from build123d import *

# Parameters (mm, degrees)
F0_W        = 127
F0_H        = 25.4
F1_DEPTH    = 3.175
F2_W        = 63.5
F2_H        = 7.9375
F3_DEPTH    = 25.4
F4_T1_DEPTH = 6.35
F5_R        = 5.08
F6_R        = 3.175
F7_DEPTH    = 25.4


# Not quite as in the source:
# - a fillet or chamfer that OpenCascade refuses, or shapes differently, is made with other operations: its cross-section is extruded or revolved along the edge and cut away or added


with BuildPart() as f1:
    # F0 (on Top) → F1 (new body, symmetric)
    with BuildSketch(Plane.XY):
        Rectangle(F0_W, F0_H)
    extrude(amount=F1_DEPTH, both=True)

    # F2 (on face) → F3 (cut)
    with BuildSketch(Plane.XY.offset(3.175)):
        with Locations((0, 8.73125)):
            Rectangle(F2_W, F2_H)
        with Locations((0, -8.73125)):
            Rectangle(F2_W, F2_H)
    extrude(amount=-F3_DEPTH, mode=Mode.SUBTRACT)

    # F4: fillet of radius 38.1 on 4 edges, made by hand

    # F4_s2 → F4_t1 (join)
    with BuildSketch(Plane.XY.offset(-3.175)):
        with BuildLine():
            ThreePointArc((-31.75, 12.7), (-20.7694028252, 6.8014320042), (-8.4726807009, 4.7625))
            Line((-8.4726807009, 4.7625), (-31.75, 4.7625))
            Line((-31.75, 4.7625), (-31.75, 12.7))
        make_face()
        with BuildLine():
            ThreePointArc((8.4726807009, 4.7625), (20.7694028252, 6.8014320042), (31.75, 12.7))
            Line((31.75, 12.7), (31.75, 4.7625))
            Line((31.75, 4.7625), (8.4726807009, 4.7625))
        make_face()
        with BuildLine():
            ThreePointArc((31.75, -12.7), (20.7694028252, -6.8014320042), (8.4726807009, -4.7625))
            Line((8.4726807009, -4.7625), (31.75, -4.7625))
            Line((31.75, -4.7625), (31.75, -12.7))
        make_face()
        with BuildLine():
            ThreePointArc((-31.75, -12.7), (-20.7694028252, -6.8014320042), (-8.4726807009, -4.7625))
            Line((-8.4726807009, -4.7625), (-31.75, -4.7625))
            Line((-31.75, -4.7625), (-31.75, -12.7))
        make_face()
    extrude(amount=F4_T1_DEPTH)

    # F5
    f5_edges = [f1.edges().sort_by_distance(p)[0] for p in [
        (-63.5, 12.7, 0),
        (-31.75, 12.7, 0),
        (-63.5, -12.7, 0),
        (-31.75, -12.7, 0),
        (31.75, -12.7, 0),
        (63.5, -12.7, 0),
        (63.5, 12.7, 0),
        (31.75, 12.7, 0),
    ]]
    fillet(f5_edges, radius=F5_R)

    # F6 (on face) → F7 (cut)
    with BuildSketch(Plane.XY.offset(3.175)):
        with Locations((-50.8, 0)):
            Circle(F6_R)
        with Locations((50.8, 0)):
            Circle(F6_R)
    extrude(amount=-F7_DEPTH, mode=Mode.SUBTRACT)


solid = f1.part
The model under review builds one solid part; all positions refer to its coordinate system, in mm. A direction names the side the tool comes from. Coordinates: 2 decimals unless noted, no trailing zeros. Loops run counter-clockwise (first coordinate to the right, second up) from the corner with the lowest first, then second, coordinate; pieces in that order, holes last.
(1) Wall thickness on L1, parallel to Y at x = 50.8, z = -1.25 (3 decimals); L2, parallel to X at y = 10.25, z = -0.25; L3, parallel to X at y = 2.5, z = -0.5: over which ranges is each line inside the solid? List them lowest first.
Determined:
L1: y = -12.7 to -3.175, 3.175 to 12.7
L2: x = -62.77 to -28.17, 28.17 to 62.77
L3: x = -63.5 to -52.76, -48.84 to 48.84, 52.76 to 63.5
(2) Tool access review of faces 1 (the cylindrical face through (-31.903, -12.468, -0.044)), 2 (the flat face through (0, 4.762, 0)), 3 (the flat face through (1, 0, -3.175)): name each direction out of +Z, -Z, +X, -X, +Y, -Y from which nothing blocks a thin tool from reaching the whole face with its end or side.
Determined:
face 1: +Z, -Z, -Y
face 2: +Z, -Z, +Y
face 3: -Z, +X, -X, +Y, -Y
(3) Consider section A-A, the plane y = 0. Give the boundary of the cut face in (x, z) (3 decimals), plus the area to 3 significant figures.
Determined:
outline: (-63.5, -3.175) - (-53.975, -3.175) - (-53.975, 3.175) - (-63.5, 3.175) - close; (-47.625, -3.175) - (47.625, -3.175) - (47.625, 3.175) - (-47.625, 3.175) - close; (53.975, -3.175) - (63.5, -3.175) - (63.5, 3.175) - (53.975, 3.175) - close
area: 726 mm2
(4) Consider section B-B, the plane z = 1.5. Give the number of separate pieces and of enclosed holes in the cut face, plus the area to 3 significant figures.
Determined:
separate pieces: 1
enclosed holes: 2
area: 2,370 mm2
(5) Insertion check: P1, Ø5.5, axis at x = 50.8, y = 0, coming from the +Z side; P2, Ø3, axis at x = -21, z = 2, coming from the -Y side; P3, Ø1.9, axis at x = 2.5, z = 1, coming from the -Y side. Each pin has a flat end and moves straight along its axis. Give the tip position at first contact, or say it passes through.
Determined:
P1: passes through
P2: stops at y = -7.44
P3: stops at y = -4.76
(6) Consider section D-D, the plane y = -9.5. Give the boundary of the cut face in (x, z) (1 decimal), plus the area to 3 significant figures.
Determined:
outline: (-63.1, -3.2) - (-26.9, -3.2) - (-26.9, 3.2) - (-63.1, 3.2) - close; (26.9, -3.2) - (63.1, -3.2) - (63.1, 3.2) - (26.9, 3.2) - close
area: 461 mm2
(7) Consider section C-C, the plane x = -50.8. Give the boundary of the cut face in (y, z) (3 decimals), plus the area to 3 significant figures.
Determined:
outline: (-12.7, -3.175) - (-3.175, -3.175) - (-3.175, 3.175) - (-12.7, 3.175) - close; (3.175, -3.175) - (12.7, -3.175) - (12.7, 3.175) - (3.175, 3.175) - close
area: 121 mm2
(8) Draft analysis for pull direction X (two halves, no side actions). For faces 4 (the cylindrical face through (61.972, 11.251, -0.044)), 5 (the flat face through (-63.5, 0, 0)), 6 (the cylindrical face through (-53.97, 0.14, 0.04)), state which applies: +X half, -X half, draft (parallel to the pull), parting line (faces both ways), or undercut.
Determined:
face 4: +X half
face 5: -X half
face 6: undercut
